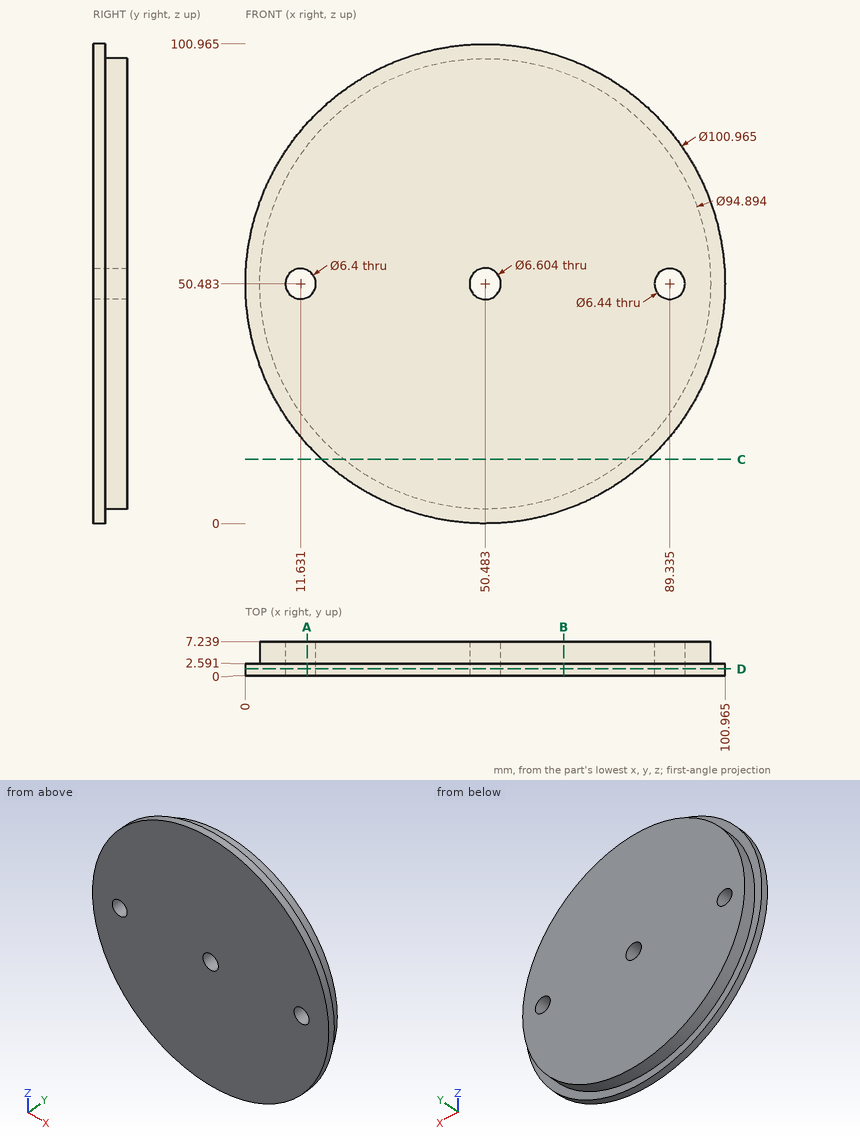
The drawing under review shows one solid part. Ordinate dimensions are in mm from its lowest x, y, z. Round coordinates to 2 decimals unless told otherwise and drop trailing zeros. Loops run counter-clockwise (first coordinate to the right, second up) from the corner with the lowest first, then second, coordinate; pieces in that order, holes last. Notation, with made-up numbers: (-35.75, -8.75) - (-8.75, -8.75) arc R24 ccw to (-8.75, 24.25) - close; hole circle Ø4 at (-16.5, -26). An arc over 180 degrees is marked (long way). Use a Markdown table: item, result. Add a question column.
Q1. Insertion check: pin 1 Ø1 at (y, z) = (3, 70.5) entering from -X (1 decimal); pin 2 Ø3 at (y, z) = (5, 20) entering from +X. Each pin has a flat end and moves straight along its axis. Give the tip position at first contact, or say it passes through.
Q2. Add section A-A (x = 13). State the section outline as (y, z) points (1 decimal), plus the area to 3 significant figures.
Q3. Add section C-C (z = 13.5). State the section outline as (x, y) points (1 decimal).
Q4. Add section D-D (y = 1.5). State the section outline as (x, z) points (1 decimal), plus the area to 3 significant figures.
Q5. Add section B-B (x = 67). State the section outline as (y, z) points.
Q6. For probe 1 along Y at (x, z) = (79, 90.5); probe 2 along X at (y, z) = (6.5, 42) (1 decimal); probe 3 along Z at (x, y) = (7, 6.75) (1 decimal), list the stretches that pass through material, from the lowest coordinate up.
Worked answers:
| question | item | result |
|---|---|---|
| 1 | pin 1 | x = 4 |
| 1 | pin 2 | x = 88.05 |
| 2 | outline | (0, 16.7) - (2.6, 16.7) - (2.6, 21.4) - (7.2, 21.4) - (7.2, 47.6) - (0, 47.6) - close; (0, 53.4) - (7.2, 53.4) - (7.2, 79.6) - (2.6, 79.6) - (2.6, 84.3) - (0, 84.3) - close |
| 2 | area | 404 mm² |
| 3 | outline | (16.1, 0) - (84.8, 0) - (84.8, 2.6) - (80.2, 2.6) - (80.2, 7.2) - (20.8, 7.2) - (20.8, 2.6) - (16.1, 2.6) - close |
| 4 | outline | circle Ø101 at (50.5, 50.5); hole circle Ø6.4 at (11.6, 50.5); hole circle Ø6.6 at (50.5, 50.5); hole circle Ø6.4 at (89.3, 50.5) |
| 4 | area | 7,910 mm² |
| 5 | outline | (0, 2.78) - (2.59, 2.78) - (2.59, 6) - (7.24, 6) - (7.24, 94.96) - (2.59, 94.96) - (2.59, 98.19) - (0, 98.19) - close |
| 6 | probe 1 | 0 to 2.59 |
| 6 | probe 2 | 3.8 to 97.2 |
| 6 | probe 3 | 31.5 to 69.5 |
